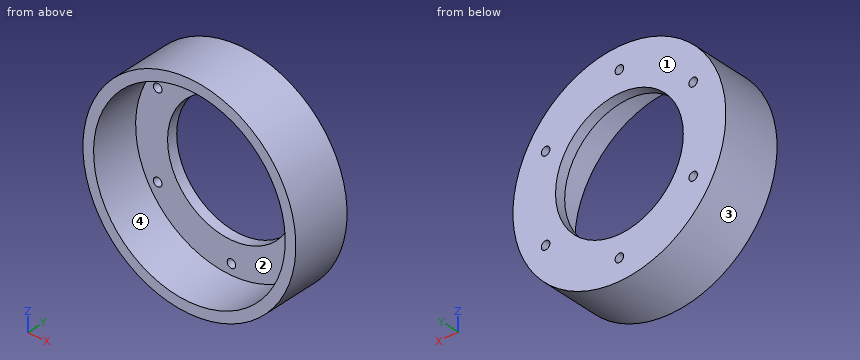
from build123d import *

# Parameters (mm, degrees)
SKETCH1_R              = 63.5
SKETCH1_R_2            = 38.1
BOSS_EXTRUDE1_DEPTH    = 35.56
SKETCH2_R              = 57.15
CUT_EXTRUDE1_DEPTH     = 29.21
F_10_CLEARANCE_HOLE1_D = 5.1054
CIRPATTERN1_COUNT      = 6


with BuildPart() as part:
    # Sketch1 → Boss-Extrude1 (new body)
    with BuildSketch(Plane(origin=(0, 0, 0), x_dir=(1, 0, 0), z_dir=(0, 1, 0))):
        with Locations(Location((0, 0, 0), (0, 0, 270))):
            Circle(SKETCH1_R)
        with Locations(Location((0, 0, 0), (0, 0, 270))):
            Circle(SKETCH1_R_2, mode=Mode.SUBTRACT)
    extrude(amount=BOSS_EXTRUDE1_DEPTH)

    # Sketch2 → Cut-Extrude1 (cut)
    with BuildSketch(Plane.XZ):
        with Locations(Location((0, 0, 0), (0, 0, 270))):
            Circle(SKETCH2_R)
    extrude(amount=-CUT_EXTRUDE1_DEPTH, mode=Mode.SUBTRACT)

    # #10 Clearance Hole1 (through all)
    with Locations(Plane(origin=(0, 35.56, 0), x_dir=(1, 0, 0), z_dir=(0, 1, 0))):
        with Locations((0, 50.8)):
            f_10_clearance_hole1 = Hole(F_10_CLEARANCE_HOLE1_D / 2)

    # CirPattern1: #10 Clearance Hole1 ×6 about axis
    cirpattern1_axis = Axis((0, 0, 0), (0, 1, 0))
    for i in range(1, CIRPATTERN1_COUNT):
        add(f_10_clearance_hole1.rotate(cirpattern1_axis, i * 360 / CIRPATTERN1_COUNT), mode=Mode.SUBTRACT)


solid = part.part
The listing builds one solid part. Answer for the finished solid, in the listing's coordinates (mm). Face numbers are marked on the shaded views. Give positions to 0.01 mm unless a question says otherwise; leave off trailing zeros. Write each loop counter-clockwise with the first axis right and the second up, starting at its lowest first coordinate (ties: lowest second). Pieces come first, ordered by that corner, then holes.
Item 1: Section C-C, the plane y = 32 is taken. Write down the section's boundary in (x, z), plus the area to 3 significant figures.
Item 2: Find the intervals of material crossed by line 1 along X through (y, z) = (7, 0); line 2 along X through (y, z) = (33, 25); line 3 along X through (y, z) = (29.5, -57), in increasing order.
Item 3: Section B-B, the plane x = 0 is taken. Write down the section's boundary in (y, z), plus the area to 3 significant figures.
Item 4: Section A-A, the plane z = 0 is taken. Write down the section's boundary in (x, y).
Item 5: Section D-D, the plane z = 25.4 is taken. Write down the section's boundary in (x, y).
Item 6: Flat-ended cylindrical pins translate along their axes: P1, Ø2, axis at x = -20.5, y = 17, coming from the -Z side; P2, Ø5, axis at y = 15, z = 28, coming from the +X side; P3, Ø4, axis at x = 43.99, z = 25.4, coming from the +Y side; P4, Ø12, axis at x = -19, y = 8.5, coming from the -Z side. Find the tip coordinate at first contact, or state that the pin passes through.
Item 7: Determine the mould class of the marked faces 1, 2, 3 and 4 for opening direction Z: released by +Z, released by -Z, zero draft, split by the parting line, or undercut.
Completed:
1. outline: circle Ø127 at (0, 0); hole circle Ø5.11 at (-43.99, -25.4); hole circle Ø5.11 at (-43.99, 25.4); hole circle Ø76.2 at (0, 0); hole circle Ø5.11 at (0, -50.8); hole circle Ø5.11 at (0, 50.8); hole circle Ø5.11 at (43.99, -25.4); hole circle Ø5.11 at (43.99, 25.4)
1. area: 7,980 mm2
2. line 1: x = -63.5 to -57.15, 57.15 to 63.5
2. line 2: x = -58.37 to -46.52, -41.47 to -28.75, 28.75 to 41.47, 46.52 to 58.37
2. line 3: x = -27.99 to 27.99
3. outline: (0, -63.5) - (35.56, -63.5) - (35.56, -53.35) - (29.21, -53.35) - (29.21, -57.15) - (0, -57.15) - close; (0, 57.15) - (29.21, 57.15) - (29.21, 53.35) - (35.56, 53.35) - (35.56, 63.5) - (0, 63.5) - close; (29.21, -48.25) - (35.56, -48.25) - (35.56, -38.1) - (29.21, -38.1) - close; (29.21, 38.1) - (35.56, 38.1) - (35.56, 48.25) - (29.21, 48.25) - close
3. area: 629 mm2
4. outline: (-63.5, 0) - (-57.15, 0) - (-57.15, 29.21) - (-38.1, 29.21) - (-38.1, 35.56) - (-63.5, 35.56) - close; (38.1, 29.21) - (57.15, 29.21) - (57.15, 0) - (63.5, 0) - (63.5, 35.56) - (38.1, 35.56) - close
5. outline: (-58.2, 0) - (-51.2, 0) - (-51.2, 29.21) - (-46.55, 29.21) - (-46.55, 35.56) - (-58.2, 35.56) - close; (-41.44, 29.21) - (-28.4, 29.21) - (-28.4, 35.56) - (-41.44, 35.56) - close; (28.4, 29.21) - (41.44, 29.21) - (41.44, 35.56) - (28.4, 35.56) - close; (46.55, 29.21) - (51.2, 29.21) - (51.2, 0) - (58.2, 0) - (58.2, 35.56) - (46.55, 35.56) - close
6. P1: stops at z = -60.43
6. P2: stops at x = 58.15
6. P3: passes through
6. P4: stops at z = -62.16
7. face 1: zero draft
7. face 2: undercut
7. face 3: split by the parting line
7. face 4: undercut
